```python
from build123d import *

# Parameters (mm, degrees)
CROQUIS1_R                     = 0.5
SALIENTE_EXTRUIR1_DEPTH        = 1.75
CROQUIS3_R                     = 4.5
CORTAR_EXTRUIR2_DEPTH          = 0.75
CORTAR_EXTRUIR3_DEPTH          = 0.75
CROQUIS5_R                     = 1.125
CORTAR_EXTRUIR4_DEPTH          = 0.5
TALADRO_ROSCADO_M1X0_251_D     = 0.75
CROQUIS8_R                     = 3
CORTAR_EXTRUIR5_DEPTH          = 0.5
TALADRO_ROSCADO_M1X0_252_D     = 0.75
TALADRO_ROSCADO_M1X0_252_DEPTH = 2
TALADRO_ROSCADO_M1X0_252_TIP   = 0.225322732


with BuildPart() as part:
    # Croquis1 → Saliente-Extruir1 (new body)
    with BuildSketch(Plane.XY):
        with BuildLine():
            ThreePointArc((8.834558852, 5.287471697), (10.400375853, 8.781625166), (10.037373186, 12.593333499))
            ThreePointArc((10.037373186, 12.593333499), (10.309088925, 13.465738911), (11.222055752, 13.428159394))
            ThreePointArc((11.222055752, 13.428159394), (13.727670201, 10.853620173), (15.654756656, 7.821674632))
            ThreePointArc((15.654756656, 7.821674632), (14.478080126, 6.085191999), (12.949014501, 4.649260976))
            ThreePointArc((12.949014501, 4.649260976), (11.201069025, 3.869086941), (9.287630024, 3.921394702))
            ThreePointArc((9.287630024, 3.921394702), (8.688101188, 4.480726783), (8.834558852, 5.287471697))
        make_face()
        with Locations((10, 5.2)):
            Circle(CROQUIS1_R, mode=Mode.SUBTRACT)
        with Locations((11.25, 12)):
            Circle(CROQUIS1_R, mode=Mode.SUBTRACT)
        with Locations((14.5, 8)):
            Circle(CROQUIS1_R, mode=Mode.SUBTRACT)
    extrude(amount=SALIENTE_EXTRUIR1_DEPTH)

    # Croquis3 → Cortar-Extruir2 (cut)
    with BuildSketch(Plane(origin=(0, 0, 0), x_dir=(-1, 0, 0), z_dir=(0, 0, -1))):
        with Locations((-10, 5.2)):
            Circle(CROQUIS3_R)
    extrude(amount=-CORTAR_EXTRUIR2_DEPTH, mode=Mode.SUBTRACT)

    # Croquis4 → Cortar-Extruir3 (cut)
    with BuildSketch(Plane(origin=(0, 0, 0), x_dir=(-1, 0, 0), z_dir=(0, 0, -1))):
        with BuildLine():
            ThreePointArc((-10.066948965, 13.181309844), (-10.613207176, 11.449681517), (-10.741563253, 9.63847766))
            ThreePointArc((-10.741563253, 9.63847766), (-10.61745437, 9.657437616), (-10.492864863, 9.672927925))
            ThreePointArc((-10.492864863, 9.672927925), (-10.410407993, 11.155791234), (-10.037373186, 12.593333499))
            ThreePointArc((-10.037373186, 12.593333499), (-9.992057529, 12.890344938), (-10.066948965, 13.181309844))
        make_face()
    extrude(amount=-CORTAR_EXTRUIR3_DEPTH, mode=Mode.SUBTRACT)

    # Croquis5 → Cortar-Extruir4 (cut)
    with BuildSketch(Plane.XY.offset(1.75)):
        with Locations((12.5, 10.25)):
            Circle(CROQUIS5_R)
    extrude(amount=-CORTAR_EXTRUIR4_DEPTH, mode=Mode.SUBTRACT)

    # Taladro roscado M1x0.251 (through all)
    with Locations(Plane.XY.offset(1.25)):
        with Locations((12.5, 10.25)):
            Hole(TALADRO_ROSCADO_M1X0_251_D / 2)

    # Croquis8 → Cortar-Extruir5 (cut)
    with BuildSketch(Plane.XY.offset(1.75)):
        with Locations((10, 5.2)):
            Circle(CROQUIS8_R)
    extrude(amount=-CORTAR_EXTRUIR5_DEPTH, mode=Mode.SUBTRACT)

    # Taladro roscado M1x0.252
    with Locations(Plane.XY.offset(1.25)):
        with Locations((11.5, 6.2)):
            Hole(TALADRO_ROSCADO_M1X0_252_D / 2, depth=TALADRO_ROSCADO_M1X0_252_DEPTH)
            with Locations((0, 0, -(TALADRO_ROSCADO_M1X0_252_DEPTH + TALADRO_ROSCADO_M1X0_252_TIP / 2))):  # 118° drill point
                Cone(0, TALADRO_ROSCADO_M1X0_252_D / 2, TALADRO_ROSCADO_M1X0_252_TIP, mode=Mode.SUBTRACT)


solid = part.part
```
Could you check a few things on this model? Use its own coordinates, in mm. A direction names the side the tool comes from. Round coordinates to 2 decimals unless told otherwise and drop trailing zeros. Loops run counter-clockwise (first coordinate to the right, second up) from the corner with the lowest first, then second, coordinate; pieces in that order, holes last.
Q1. I want a section at A-A (y = 10.25). Write out the boundary of the cut face in (x, z) (3 decimals).
Q2. I want a section at C-C (x = 11.5). Write out the boundary of the cut face in (y, z) (3 decimals), and give its area (3 significant figures).
Q3. I want a section at B-B (z = 1.15). Write out the boundary of the cut face in (x, y) (3 decimals), and give its area (3 significant figures).
Q4. Thinking about a two-plate mould opening in X: for faces 6 (the flat face through (12, 11, 1.25)), 7 (the flat face through (13, 9, 1.75)), 8 (the cylindrical face through (11.228, 3.874, 0.996)), which applies, pulls with the +X half, pulls with the -X half, needs draft (parallel to the pull), parting line crosses it, or undercut?
Q5. I want a section at D-D (x = 12.5). Write out the boundary of the cut face in (y, z) (3 decimals), and give its area (3 significant figures).
Q6. For P1, Ø1.5, axis at x = 13.5, y = 5.5, coming from the -Z side; P2, Ø3.5, axis at x = 10, y = 5.5, coming from the +Z side, each with a flat end and sliding along its axis, tell me the tip position at first contact or that it passes through.
Q7. On a 3-axis mill with a long thin cutter (end or side, diameter ignored), from which of +Z, -Z, +X, -X, +Y, -Y can I reach the whole of each face in a straight line? I mean faces 1 (the cylindrical face through (13.7, 10.89, 0.86)), 2 (the cylindrical face through (13.019, 9.252, 1.504)), 3 (the flat face through (13, 10, 0)), 4 (the cylindrical face through (12.4, 7, 1.5)), 5 (the cylindrical face through (13.125, 8.438, 0.37)). Say none if no direction works.
Q8. Please list where these lines run through material, in increasing order: L1, parallel to Z at x = 10.5, y = 11.75; L2, parallel to Y at x = 14.5, z = 1.15; L3, parallel to X at y = 5.2, z = 0.95.
Answer below:
1. outline: (10.496, 0.75) - (10.746, 0.75) - (10.746, 0) - (12.125, 0) - (12.125, 1.25) - (11.375, 1.25) - (11.375, 1.75) - (10.496, 1.75) - close; (12.875, 0) - (14.184, 0) - (14.184, 1.75) - (13.625, 1.75) - (13.625, 1.25) - (12.875, 1.25) - close
2. outline: (3.94, 0.75) - (5.825, 0.75) - (5.825, 1.25) - (3.94, 1.25) - close; (6.575, 0.75) - (9.443, 0.75) - (9.443, 0) - (11.567, 0) - (11.567, 1.75) - (10.765, 1.75) - (10.765, 1.25) - (9.735, 1.25) - (9.735, 1.75) - (7.798, 1.75) - (7.798, 1.25) - (6.575, 1.25) - close; (12.433, 0) - (13.191, 0) - (13.191, 1.75) - (12.433, 1.75) - close
2. area: 7.73 mm2
3. outline: (8.835, 5.287) arc R0.855 ccw to (9.288, 3.921) arc R4.317 ccw to (12.949, 4.649) arc R9.5 ccw to (15.655, 7.822) arc R17.5 ccw to (11.222, 13.428) arc R0.75 ccw to (10.037, 12.593) arc R7.5 cw to start; hole circle Ø1 at (10, 5.2); hole circle Ø1 at (11.25, 12); hole circle Ø0.75 at (11.5, 6.2); hole circle Ø0.75 at (12.5, 10.25); hole circle Ø1 at (14.5, 8)
3. area: 35.0 mm2
4. face 6: undercut
4. face 7: needs draft
4. face 8: parting line crosses it
5. outline: (4.354, 0.75) - (8.942, 0.75) - (8.942, 0) - (9.875, 0) - (9.875, 1.25) - (9.125, 1.25) - (9.125, 1.75) - (6.858, 1.75) - (6.858, 1.25) - (4.354, 1.25) - close; (10.625, 0) - (12.247, 0) - (12.247, 1.75) - (11.375, 1.75) - (11.375, 1.25) - (10.625, 1.25) - close
5. area: 7.06 mm2
6. P1: stops at z = 0.75
6. P2: stops at z = 1.25
7. face 1: +Z, -Z, +X, +Y
7. face 2: +Z
7. face 3: -Z, +X, -X, +Y, -Y
7. face 4: +Z, -X
7. face 5: -Z, -X, -Y
8. L1: z = 0.75 to 1.75
8. L2: y = 6.11 to 7.5, 8.5 to 9.8
8. L3: x = 8.77 to 9.5, 10.5 to 13.62
